The drawing under review shows one solid part. Ordinate dimensions are in mm from its lowest x, y, z. A direction names the side the tool comes from. Coordinates: 2 decimals unless noted, no trailing zeros. Order: outer loops, then holes, each group sorted by start corner. A loop starts at its lowest first (then second) coordinate and runs counter-clockwise, first axis right, second up. Notation, with made-up numbers: (14, -15.75) - (33, -15.75) arc R13 ccw to (33, 0.25) - close; hole circle Ø3 at (-39, 35.5). An arc over 180 degrees is marked (long way). Answer in a Markdown table with one row per item.
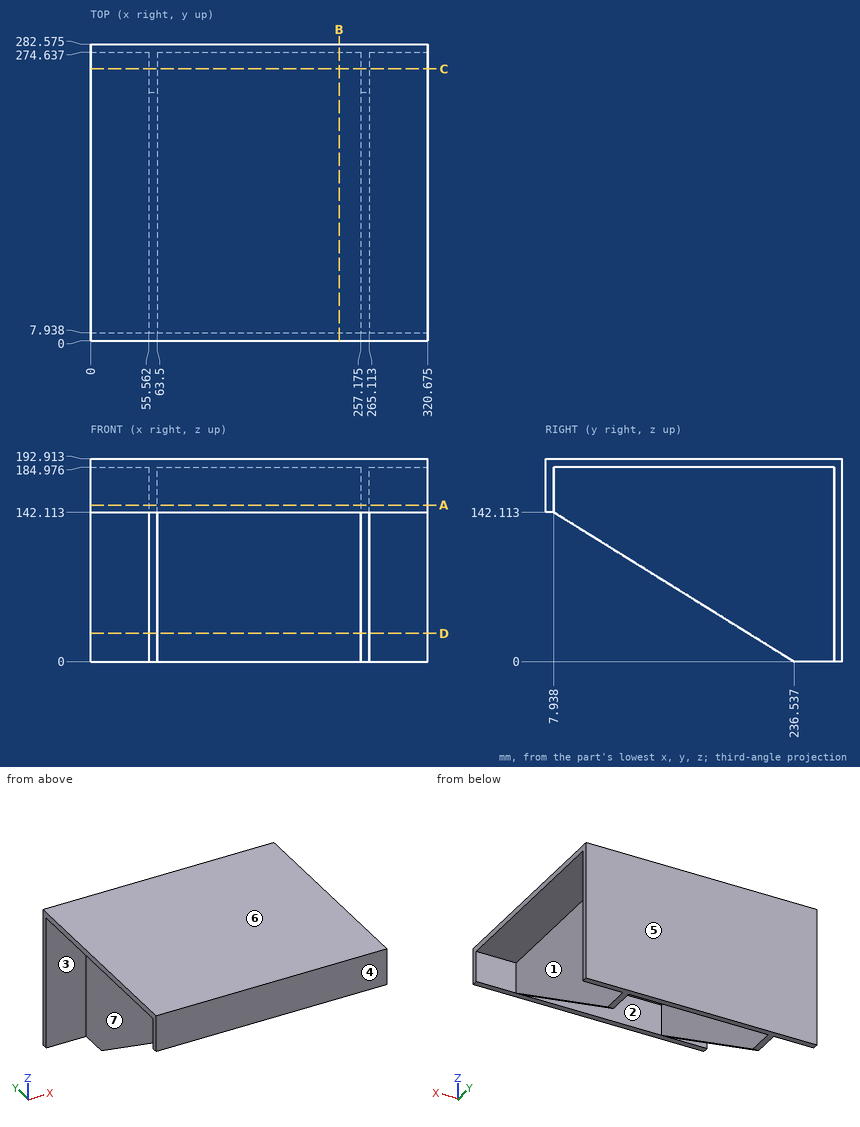
Item 1: We need section B-B, the plane x = 236.5. Write out the cut boundary in (y, z) (1 decimal).
Check values:
| item | result |
|---|---|
| outline | (0, 142.1) - (7.9, 142.1) - (7.9, 185) - (274.6, 185) - (274.6, 0) - (282.6, 0) - (282.6, 192.9) - (0, 192.9) - close |
Item 2: We need section C-C, the plane y = 259. Write out the cut boundary in (x, z) (1 decimal).
Check values:
| item | result |
|---|---|
| outline | (0, 185) - (55.6, 185) - (55.6, 0) - (63.5, 0) - (63.5, 185) - (257.2, 185) - (257.2, 0) - (265.1, 0) - (265.1, 185) - (320.7, 185) - (320.7, 192.9) - (0, 192.9) - close |
Item 3: We need section D-D, the plane z = 27. Write out the cut boundary in (x, y) (1 decimal), then the cut area to 3 significant figures.
Check values:
| item | result |
|---|---|
| outline | (0, 274.6) - (55.6, 274.6) - (55.6, 193.1) - (63.5, 193.1) - (63.5, 274.6) - (257.2, 274.6) - (257.2, 193.1) - (265.1, 193.1) - (265.1, 274.6) - (320.7, 274.6) - (320.7, 282.6) - (0, 282.6) - close |
| area | 3,840 mm^2 |
Item 4: To check wall thickness, follow line 1 (X direction, y = 58.5, z = 183) (1 decimal); line 2 (Y direction, x = 266, z = 166) (1 decimal); line 3 (Y direction, x = 267.5, z = 68.5) (1 decimal). State the ranges of each line that lie inside material, in increasing order. Write a range as from..to.
Check values:
| item | result |
|---|---|
| line 1 | 55.6..63.5, 257.2..265.1 |
| line 2 | 0..7.9, 274.6..282.6 |
| line 3 | 274.6..282.6 |
Item 5: We need section A-A, the plane z = 149. Write out the cut boundary in (x, y) (1 decimal).
Check values:
| item | result |
|---|---|
| outline | (0, 0) - (320.7, 0) - (320.7, 7.9) - (265.1, 7.9) - (265.1, 274.6) - (320.7, 274.6) - (320.7, 282.6) - (0, 282.6) - (0, 274.6) - (55.6, 274.6) - (55.6, 7.9) - (0, 7.9) - close; hole (63.5, 7.9) - (257.2, 7.9) - (257.2, 274.6) - (63.5, 274.6) - close |
Item 6: Clearance check with flat-ended pins moving along their axes: pin 1 Ø5 at (x, z) = (229.5, 117.5) entering from -Y; pin 2 Ø10 at (y, z) = (209, 170) entering from +X; pin 3 Ø2 at (y, z) = (119.5, 112) entering from -X. State where each tip first meets the part, or that it passes through.
Check values:
| item | result |
|---|---|
| pin 1 | y = 274.64 |
| pin 2 | x = 265.11 |
| pin 3 | x = 55.56 |
Item 7: Mouldability with a two-part tool opening along Y and no side actions: class the marked faces 4, 5, 6 and 7 as +Y half, -Y half, draft (parallel to the pull), parting line (faces both ways), or undercut.
Check values:
| item | result |
|---|---|
| face 4 | -Y half |
| face 5 | +Y half |
| face 6 | draft |
| face 7 | undercut |
Item 8: Tool access review of the marked faces 1, 2 and 3: name each direction out of +Z, -Z, +X, -X, +Y, -Y from which nothing blocks a thin tool from reaching the whole face with its end or side.
Check values:
| item | result |
|---|---|
| face 1 | -Z, +X |
| face 2 | -Z |
| face 3 | -Z, -X |
